The model under review builds one solid part; all positions refer to its coordinate system, in mm. Coordinates: 2 decimals unless noted, no trailing zeros. Order: outer loops, then holes, each group sorted by start corner. A loop starts at its lowest first (then second) coordinate and runs counter-clockwise, first axis right, second up. Notation, with made-up numbers: (61, -20) -> (88, -20) arc R24 ccw to (88, 19) -> close; hole circle Ø7 at (43, 72). An arc over 180 degrees is marked (long way). Answer as CSV lines item,"result". Start each with the question number.
from build123d import *

# Parameters (mm, degrees)
SZKIC1_R                    = 20
DODANIE_WYCI_GNI_CIE1_DEPTH = 12
SZKIC4_R                    = 9
WYTNIJ_WYCI_GNI_CIE1_DEPTH  = 12
ZAOKR_GLENIE1_R             = 0.5


with BuildPart() as part:
    # Szkic1 → Dodanie-wyciągnięcie1 (new body)
    with BuildSketch(Plane.XY):
        Circle(SZKIC1_R)
    extrude(amount=DODANIE_WYCI_GNI_CIE1_DEPTH)

    # Szkic4 → Wytnij-wyciągnięcie1 (cut)
    with BuildSketch(Plane(origin=(0, 0, 0), x_dir=(-1, 0, 0), z_dir=(0, 0, -1))):
        Circle(SZKIC4_R)
    extrude(amount=-WYTNIJ_WYCI_GNI_CIE1_DEPTH, mode=Mode.SUBTRACT)

    # Zaokrąglenie1
    zaokr_glenie1_edges = [part.edges().sort_by_distance(p)[0] for p in [
        (-20, 0, 0),
        (-20, 0, 12),
        (9, 0, 12),
        (9, 0, 0),
    ]]
    fillet(zaokr_glenie1_edges, radius=ZAOKR_GLENIE1_R)


solid = part.part
1) Wall thickness on L1, parallel to Y at x = 0, z = 7.5; L2, parallel to Y at x = -3.5, z = 2.75; L3, parallel to X at y = 10.5, z = 3.25: over which ranges is each line inside the solid? List them lowest first. Write a range as [from, to].
2) Mouldability with a two-part tool opening along X and no side actions: class faces 1 (the face through (-4.336, -19.524, 5.923)), 2 (the face through (4, 9, 12)), 3 (the face through (1.172, 8.923, 5.923)) as released by +X, released by -X, zero draft, split by the parting line, or undercut.
3) Consider section A-A (y = 0). Give the boundary of the cut face in (x, z), plus the area to 3 significant figures.
4) Consider section C-C (z = 3.75). Give the boundary of the cut face in (x, y).
5) Insertion check: pin 1 Ø1.5 at (y, z) = (-9, 8) entering from -X; pin 2 Ø6 at (x, z) = (12, 3) entering from -Y; pin 3 Ø6 at (y, z) = (11, 5.5) entering from -X. Each pin has a flat end and moves straight along its axis. Give the tip position at first contact, or say it passes through.
Result:
1,L1,"[-20, -9], [9, 20]"
1,L2,"[-19.69, -8.29], [8.29, 19.69]"
1,L3,"[-17.02, 17.02]"
2,face 1,"split by the parting line"
2,face 2,"zero draft"
2,face 3,"undercut"
3,outline,"(-20, 0.5) arc R0.5 ccw to (-19.5, 0) -> (-9.5, 0) arc R0.5 ccw to (-9, 0.5) -> (-9, 11.5) arc R0.5 ccw to (-9.5, 12) -> (-19.5, 12) arc R0.5 ccw to (-20, 11.5) -> close; (9, 0.5) arc R0.5 ccw to (9.5, 0) -> (19.5, 0) arc R0.5 ccw to (20, 0.5) -> (20, 11.5) arc R0.5 ccw to (19.5, 12) -> (9.5, 12) arc R0.5 ccw to (9, 11.5) -> close"
3,area,"264 mm2"
4,outline,"circle Ø40 at (0, 0); hole circle Ø18 at (0, 0)"
5,pin 1,"x = -18.22"
5,pin 2,"y = -17.86"
5,pin 3,"x = -18.33"
